Can you work these out from the model? Positions are in its coordinate system, mm. Face numbers are marked on the shaded views. A direction names the side the tool comes from. Round coordinates to 2 decimals unless told otherwise and drop trailing zeros. Order: outer loops, then holes, each group sorted by start corner. A loop starts at its lowest first (then second) coordinate and runs counter-clockwise, first axis right, second up. Notation, with made-up numbers: M 47.25,58.25 L 74.25,58.25 A18 cw 74.25,70.25 Z; hole C 14.5,-18.75 d11. An arc over 180 degrees is marked long. One line per question, with ' | ' between items.
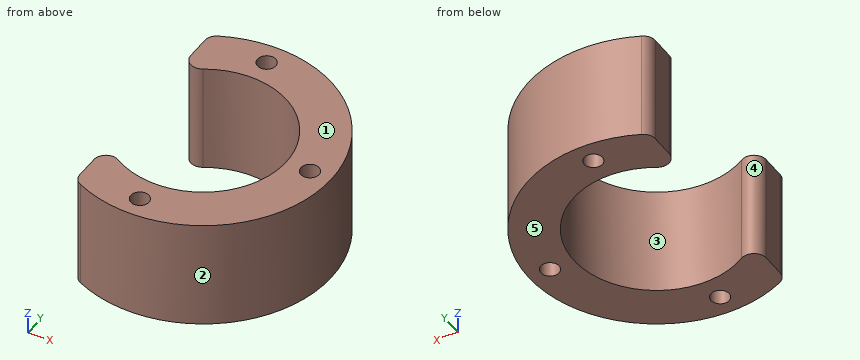
```python
from build123d import *

# Parameters (mm, degrees)
SKETCH_1_R          = 21
EXTRUDE_1_DEPTH     = 18
SKETCH_2_R          = 1.5
SKETCH_2_R_2        = 13.6
CUT_EXTRUDE_1_DEPTH = 25
SKETCH_4_W          = 14.155551169
SKETCH_4_H          = 37.805917944
CUT_EXTRUDE_2_DEPTH = 25
FILLET_1_R          = 2


with BuildPart() as part:
    # 草图1 → 凸台-拉伸1 (new body)
    with BuildSketch(Plane.XY):
        Circle(SKETCH_1_R)
    extrude(amount=EXTRUDE_1_DEPTH)

    # 草图2 → 切除-拉伸1 (cut)
    with BuildSketch(Plane.XY.offset(18)):
        with Locations((-17.5, 0)):
            Circle(SKETCH_2_R)
        Circle(SKETCH_2_R_2)
        with Locations((0, 17.5)):
            Circle(SKETCH_2_R)
        with Locations((17.5, 0)):
            Circle(SKETCH_2_R)
        with Locations((0, -17.5)):
            Circle(SKETCH_2_R)
    extrude(amount=-CUT_EXTRUDE_1_DEPTH, mode=Mode.SUBTRACT)

    # 草图4 → 切除-拉伸2 (cut)
    with BuildSketch(Plane(origin=(0, 0, 0), x_dir=(-1, 0, 0), z_dir=(0, 0, -1))):
        with Locations((17.077775585, -0.436773659)):
            Rectangle(SKETCH_4_W, SKETCH_4_H)
    extrude(amount=-CUT_EXTRUDE_2_DEPTH, mode=Mode.SUBTRACT)

    # 圆角1
    fillet_1_edges = [part.edges().sort_by_distance(p)[0] for p in [
        (-10, -9.217374897, 9),
        (-10, 9.217374897, 9),
        (-10, -18.466185313, 9),
        (-10, 18.466185313, 9),
    ]]
    fillet(fillet_1_edges, radius=FILLET_1_R)


solid = part.part
```
(1) If we section it at A-A on x = 0: Please give me the cut outline in (y, z), plus the area to 3 significant figures.
Final values:
outline: M -21,0 L -19,0 L -19,18 L -21,18 Z; M -16,0 L -13.6,0 L -13.6,18 L -16,18 Z; M 13.6,0 L 16,0 L 16,18 L 13.6,18 Z; M 19,0 L 21,0 L 21,18 L 19,18 Z | area: 158 mm^2
(2) If we section it at D-D on z = 13.5: Please give me the cut outline in (x, y), plus the area to 3 significant figures.
Final values:
outline: M -10,-17.23 A2 ccw -8.84,-19.05 A21 ccw long -8.84,19.05 A2 ccw -10,17.23 L -10,13.39 A2 ccw -6.97,11.68 A13.6 cw long -6.97,-11.68 A2 ccw -10,-13.39 Z; hole C 0,-17.5 d3; hole C 0,17.5 d3; hole C 17.5,0 d3 | area: 532 mm^2
(3) If we section it at B-B on y = 0: Please give me the cut outline in (x, z).
Final values:
outline: M 13.6,0 L 16,0 L 16,18 L 13.6,18 Z; M 19,0 L 21,0 L 21,18 L 19,18 Z
(4) Please list where these lines run through material, in increasing order: probe 1 along Y at (x, z) = (0, 6.5); probe 2 along Y at (x, z) = (-4, 8.5); probe 3 along Y at (x, z) = (6.5, 6.75). Write a range as [from, to].
Final values:
probe 1: [-21, -19], [-16, -13.6], [13.6, 16], [19, 21] | probe 2: [-20.62, -13], [13, 20.62] | probe 3: [-19.97, -11.95], [11.95, 19.97]
(5) If we section it at C-C on x = 17.5: Please give me the cut outline in (y, z), plus the area to 3 significant figures.
Final values:
outline: M -11.61,0 L -1.5,0 L -1.5,18 L -11.61,18 Z; M 1.5,0 L 11.61,0 L 11.61,18 L 1.5,18 Z | area: 364 mm^2
(6) Thinking about a two-plate mould opening in Y: for the marked faces 1, 2 and 3, which applies, released by +Y, released by -Y, zero draft, split by the parting line, or undercut?
Final values:
face 1: zero draft | face 2: split by the parting line | face 3: undercut
(7) On a 3-axis mill with a long thin cutter (end or side, diameter ignored), from which of +Z, -Z, +X, -X, +Y, -Y can I reach the whole of each face in a straight line? I mean the marked faces 4 and 5. Say none if no direction works.
Final values:
face 4: +Z, -Z | face 5: -Z, +X, -X, +Y, -Y
(8) Will these pins go through, and if not, where does the flat tip stop? pin 1 Ø5 at (x, y) = (7, -6) entering from -Z; pin 2 Ø4 at (x, z) = (5, 12) entering from +Y; pin 3 Ø6 at (y, z) = (-10, 4) entering from -X; pin 4 Ø3 at (x, z) = (-4.5, 16) entering from -Y.
Final values:
pin 1: through | pin 2: y = 20.78 | pin 3: x = -9.96 | pin 4: y = -20.78
